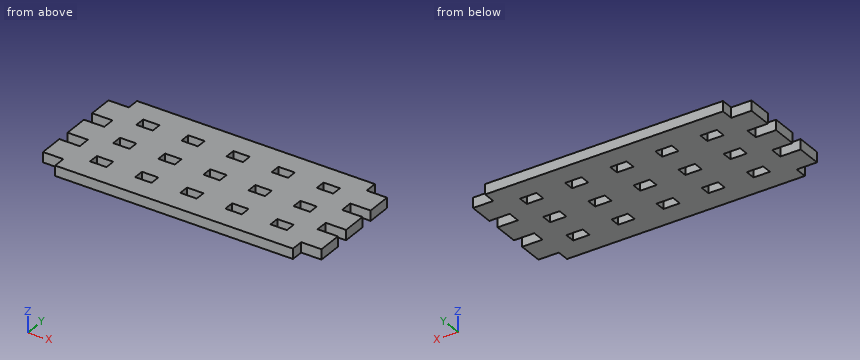
```python
from build123d import *

# Parameters (mm, degrees)
MODEL_W             = 20
MODEL_H             = 12.4
BOSS_EXTRUDE1_DEPTH = 12.4


with BuildPart() as part:
    # Model → Boss-Extrude1 (new body)
    with BuildSketch(Plane.XY):
        Polygon((0, 135), (0, 150), (290, 150), (290, 135), (314.8, 135), (314.8, 105), (290, 105), (290, 90), (314.8, 90), (314.8, 60), (290, 60), (290, 45), (314.8, 45), (314.8, 15), (290, 15), (290, 0), (0, 0), (0, 15), (-24.8, 15), (-24.8, 45), (0, 45), (0, 60), (-24.8, 60), (-24.8, 90), (0, 90), (0, 105), (-24.8, 105), (-24.8, 135), align=None)
        with Locations((200, 117.4)):
            Rectangle(MODEL_W, MODEL_H, mode=Mode.SUBTRACT)
        with Locations((145, 117.4)):
            Rectangle(MODEL_W, MODEL_H, mode=Mode.SUBTRACT)
        with Locations((255, 117.4)):
            Rectangle(MODEL_W, MODEL_H, mode=Mode.SUBTRACT)
        with Locations((200, 75)):
            Rectangle(MODEL_W, MODEL_H, mode=Mode.SUBTRACT)
        with Locations((255, 75)):
            Rectangle(MODEL_W, MODEL_H, mode=Mode.SUBTRACT)
        with Locations((200, 32.6)):
            Rectangle(MODEL_W, MODEL_H, mode=Mode.SUBTRACT)
        with Locations((255, 32.6)):
            Rectangle(MODEL_W, MODEL_H, mode=Mode.SUBTRACT)
        with Locations((145, 75)):
            Rectangle(MODEL_W, MODEL_H, mode=Mode.SUBTRACT)
        with Locations((145, 32.6)):
            Rectangle(MODEL_W, MODEL_H, mode=Mode.SUBTRACT)
        with Locations((90, 117.4)):
            Rectangle(MODEL_W, MODEL_H, mode=Mode.SUBTRACT)
        with Locations((35, 117.4)):
            Rectangle(MODEL_W, MODEL_H, mode=Mode.SUBTRACT)
        with Locations((90, 75)):
            Rectangle(MODEL_W, MODEL_H, mode=Mode.SUBTRACT)
        with Locations((35, 75)):
            Rectangle(MODEL_W, MODEL_H, mode=Mode.SUBTRACT)
        with Locations((90, 32.6)):
            Rectangle(MODEL_W, MODEL_H, mode=Mode.SUBTRACT)
        with Locations((35, 32.6)):
            Rectangle(MODEL_W, MODEL_H, mode=Mode.SUBTRACT)
    extrude(amount=BOSS_EXTRUDE1_DEPTH)


solid = part.part
```
Geometry: final body of the model. Coordinates: model frame, mm. Coordinates: 2 decimals unless noted, no trailing zeros. Order: outer loops, then holes, each group sorted by start corner. A loop starts at its lowest first (then second) coordinate and runs counter-clockwise, first axis right, second up.
Item 1: Section query B-B (x = 87.5). Output: boundary loops of the cut face in (y, z).
Answer:
outline: (0, 0) - (26.4, 0) - (26.4, 12.4) - (0, 12.4) - close; (38.8, 0) - (68.8, 0) - (68.8, 12.4) - (38.8, 12.4) - close; (81.2, 0) - (111.2, 0) - (111.2, 12.4) - (81.2, 12.4) - close; (123.6, 0) - (150, 0) - (150, 12.4) - (123.6, 12.4) - close
Item 2: Section query C-C (z = 4.5). State how many separate pieces and enclosed holes the cut face has, then the cut area to 3 significant figures.
Answer:
separate pieces: 1
enclosed holes: 15
area: 44,200 mm2
Item 3: Section query D-D (y = 96). Output: boundary loops of the cut face in (x, z), then the cut area to 3 significant figures.
Answer:
outline: (0, 0) - (290, 0) - (290, 12.4) - (0, 12.4) - close
area: 3,600 mm2
Item 4: Material intervals for line 1 along X through (y, z) = (27, 3.5); line 2 along Y through (x, z) = (209, 0.5); line 3 along X through (y, z) = (99, 0.5), sorted ascending.
Answer:
line 1: x = -24.8 to 25, 45 to 80, 100 to 135, 155 to 190, 210 to 245, 265 to 314.8
line 2: y = 0 to 26.4, 38.8 to 68.8, 81.2 to 111.2, 123.6 to 150
line 3: x = 0 to 290
Item 5: Contact query for flat-ended pins moving along their axis: P1, Ø3.5, axis at x = 305.5, z = 9, coming from the +Y side; P2, Ø3.5, axis at x = 299.5, z = 3, coming from the -Y side; P3, Ø3.5, axis at y = 97.5, z = 7.5, coming from the -X side. Output: stop coordinate, or through.
Answer:
P1: stops at y = 135
P2: stops at y = 15
P3: stops at x = 0
Item 6: Section query A-A (y = 30). Output: boundary loops of the cut face in (x, z).
Answer:
outline: (-24.8, 0) - (25, 0) - (25, 12.4) - (-24.8, 12.4) - close; (45, 0) - (80, 0) - (80, 12.4) - (45, 12.4) - close; (100, 0) - (135, 0) - (135, 12.4) - (100, 12.4) - close; (155, 0) - (190, 0) - (190, 12.4) - (155, 12.4) - close; (210, 0) - (245, 0) - (245, 12.4) - (210, 12.4) - close; (265, 0) - (314.8, 0) - (314.8, 12.4) - (265, 12.4) - close
